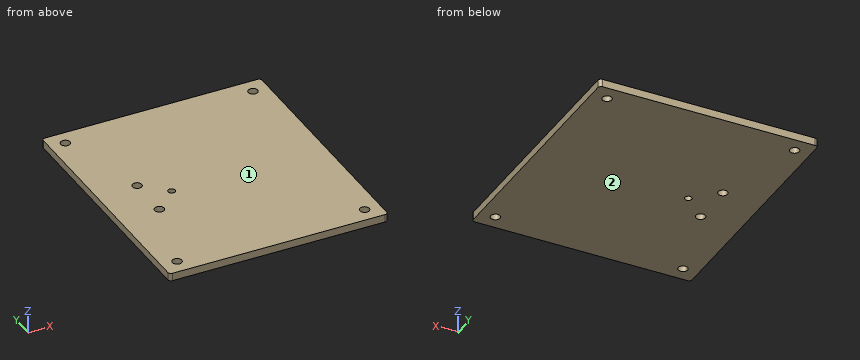
```python
from build123d import *

# Parameters (mm, degrees)
MODEL_W             = 140
MODEL_H             = 160
MODEL_R             = 3
MODEL_R_2           = 2.25
BOSS_EXTRUDE1_DEPTH = 5
FILLET1_R           = 2


with BuildPart() as part:
    # Model → Boss-Extrude1 (new body)
    with BuildSketch(Plane.XY):
        with Locations((70, 80)):
            Rectangle(MODEL_W, MODEL_H)
        with Locations((26, 91.5)):
            Circle(MODEL_R, mode=Mode.SUBTRACT)
        with Locations((10, 150)):
            Circle(MODEL_R, mode=Mode.SUBTRACT)
        with Locations((130, 10)):
            Circle(MODEL_R, mode=Mode.SUBTRACT)
        with Locations((10, 10)):
            Circle(MODEL_R, mode=Mode.SUBTRACT)
        with Locations((130, 150)):
            Circle(MODEL_R, mode=Mode.SUBTRACT)
        with Locations((26, 63.5)):
            Circle(MODEL_R, mode=Mode.SUBTRACT)
        with Locations((41, 77.5)):
            Circle(MODEL_R_2, mode=Mode.SUBTRACT)
    extrude(amount=BOSS_EXTRUDE1_DEPTH)

    # Fillet1
    fillet1_edges = [part.edges().sort_by_distance(p)[0] for p in [
        (0, 0, 2.5),
        (0, 160, 2.5),
        (140, 160, 2.5),
        (140, 0, 2.5),
    ]]
    fillet(fillet1_edges, radius=FILLET1_R)


solid = part.part
```
Input: part model. Units: mm. Frame: model coordinates. Face numbers are marked on the shaded views. Round coordinates to 2 decimals unless told otherwise and drop trailing zeros. Loops run counter-clockwise (first coordinate to the right, second up) from the corner with the lowest first, then second, coordinate; pieces in that order, holes last. Notation, with made-up numbers: (15.25, -37) -> (28.25, -37) arc R18 cw to (28.25, -26) -> close; hole circle Ø5 at (37.25, 11.25). An arc over 180 degrees is marked (long way). Use one line per item in the form item = value. Start each with the question number.
Item 1: Section query C-C on y = 10. Return the cut outline in (x, z), then the cut area to 3 significant figures.
Item 2: Material intervals for L1, parallel to X at y = 150, z = 2.6; L2, parallel to Y at x = 130, z = 2.4; L3, parallel to Y at x = 26, z = 3.5, sorted ascending. Write a range as from..to.
Item 3: Section query B-B on x = 10. Return the cut outline in (y, z), then the cut area to 3 significant figures.
Item 4: Section query A-A on y = 77.5. Return the cut outline in (x, z).
Item 5: Contact query for a flat-ended pin moving along its axis: pin 1 Ø5 at (x, y) = (10, 10) entering from -Z. Output: stop coordinate, or through.
Item 6: Section query D-D on x = 41. Return the cut outline in (y, z), then the cut area to 4 significant figures.
Item 7: Mould query, pull axis Z, two halves, no side actions, for the marked faces 1 and 2. Classes: pulls with the +Z half, pulls with the -Z half, needs draft (parallel to the pull), parting line crosses it, or undercut.
Ans:
q1.outline = (0, 0) -> (7, 0) -> (7, 5) -> (0, 5) -> close; (13, 0) -> (127, 0) -> (127, 5) -> (13, 5) -> close; (133, 0) -> (140, 0) -> (140, 5) -> (133, 5) -> close
q1.area = 640 mm^2
q2.L1 = 0..7, 13..127, 133..140
q2.L2 = 0..7, 13..147, 153..160
q2.L3 = 0..60.5, 66.5..88.5, 94.5..160
q3.outline = (0, 0) -> (7, 0) -> (7, 5) -> (0, 5) -> close; (13, 0) -> (147, 0) -> (147, 5) -> (13, 5) -> close; (153, 0) -> (160, 0) -> (160, 5) -> (153, 5) -> close
q3.area = 740 mm^2
q4.outline = (0, 0) -> (38.75, 0) -> (38.75, 5) -> (0, 5) -> close; (43.25, 0) -> (140, 0) -> (140, 5) -> (43.25, 5) -> close
q5.pin_1 = through
q6.outline = (0, 0) -> (75.25, 0) -> (75.25, 5) -> (0, 5) -> close; (79.75, 0) -> (160, 0) -> (160, 5) -> (79.75, 5) -> close
q6.area = 777.5 mm^2
q7.face_1 = pulls with the +Z half
q7.face_2 = pulls with the -Z half
